The listing builds one solid part. Answer for the finished solid, in the listing's coordinates (mm). A direction names the side the tool comes from. Coordinates: 2 decimals unless noted, no trailing zeros. Loops run counter-clockwise (first coordinate to the right, second up) from the corner with the lowest first, then second, coordinate; pieces in that order, holes last. Notation, with made-up numbers: (65, -3.5) - (116, -3.5) arc R18 ccw to (116, 27.5) - close; hole circle Ø7 at (25.25, -4.75). An arc over 180 degrees is marked (long way). Write each question's results on one line, items separated by ' | '. Start each with the question number.
(1) Find section D-D on x = 4. Determine the outline of the cut face in (y, z).
(2) Find section C-C on x = 0. Determine the outline of the cut face in (y, z), then the cut area to 3 significant figures.
(3) Find section A-A on z = 6.5. Determine the outline of the cut face in (x, y).
(4) Consider line 1 (X direction, y = 9.75, z = 3.25); line 2 (Z direction, x = 2.5, y = -5.5); line 3 (Y direction, x = -9.5, z = 3.75). Determine where each line is inside the solid, lowest interval first. Write a range as from..to.
(5) Given pin 1 Ø6 at (y, z) = (7, 3.5) entering from +X; pin 2 Ø1.5 at (x, z) = (3, 5) entering from -Y; pin 3 Ø2.5 at (x, z) = (7, 5.5) entering from +Y, each flat-ended and moving along its own axis, determine where each tip first touches the part or whether it passes through.
(6) For faces 4 (the flat face through (-8, -0.585, 5)), 5 (the flat face through (0, -10.589, 3)), 6 (the cylindrical face through (2.307, -4.436, 7.395)), 7 (the flat face through (0.66, -8, 5)), 8 (the flat face through (-10, 0, 3)), determine the directions among +Z, -Z, +X, -X, +Y, -Y from which every point of the face is accessible in a straight line to the end or side of a thin tool.
(7) Determine the mould class of faces 1 (the cylindrical face through (11.923, 3.755, -0.986)), 2 (the flat face through (-8, 0.585, 5)), 3 (the flat face through (-0.66, 8, 5)) for opening direction X: released by +X, released by -X, zero draft, split by the parting line, or undercut.
from build123d import *

# Parameters (mm, degrees)
F0_R     = 5
F2_DEPTH = 15
F1_W     = 9.3396854261
F1_H     = 1.1709111985
F1_W_2   = 1.3206291478
F1_H_2   = 10.0037873136
F3_DEPTH = 12
F4_SIZE  = 4.99999
F5_R     = 12.5
F6_DEPTH = 2


# Not quite as in the source:
# - a fillet or chamfer is up to 0.001 mm smaller than in the source, because OpenCascade refuses the exact size


with BuildPart() as f2:
    # F0 (on Top) → F2 (new body)
    with BuildSketch(Plane.XY):
        Circle(F0_R)
    extrude(amount=F2_DEPTH)

    # F1 (on Top) → F3 (join)
    with BuildSketch(Plane.XY):
        with Locations((5.330157287, 0)):
            Rectangle(F1_W, F1_H)
        with Locations((-5.330157287, 0)):
            Rectangle(F1_W, F1_H)
        with Locations((0, 5.587349256)):
            Rectangle(F1_W_2, F1_H_2)
        with Locations((0, -5.587349256)):
            Rectangle(F1_W_2, F1_H_2)
    extrude(amount=F3_DEPTH)

    # F4 (size 5 in the source; OpenCascade refuses exactly that, so slightly less here)
    f4_edges = [f2.edges().sort_by_distance(p)[0] for p in [
        (0, 10.589243, 12),
        (10, 0, 12),
        (0, -10.589243, 12),
        (-10, 0, 12),
    ]]
    chamfer(f4_edges, length=F4_SIZE)

    # F5 (on Top) → F6 (join)
    with BuildSketch(Plane.XY):
        Circle(F5_R)
    extrude(amount=-F6_DEPTH)


solid = f2.part
Values:
1) outline: (-11.84, -2) - (11.84, -2) - (11.84, 0) - (3, 0) - (3, 15) - (-3, 15) - (-3, 0) - (-11.84, 0) - close
2) outline: (-12.5, -2) - (12.5, -2) - (12.5, 0) - (10.59, 0) - (10.59, 7) - (5.59, 12) - (5, 12) - (5, 15) - (-5, 15) - (-5, 12) - (-5.59, 12) - (-10.59, 7) - (-10.59, 0) - (-12.5, 0) - close | area: 309 mm²
3) outline: (-10, -0.59) - (-4.97, -0.59) arc R5 ccw to (-0.66, -4.96) - (-0.66, -10.59) - (0.66, -10.59) - (0.66, -4.96) arc R5 ccw to (4.97, -0.59) - (10, -0.59) - (10, 0.59) - (4.97, 0.59) arc R5 ccw to (0.66, 4.96) - (0.66, 10.59) - (-0.66, 10.59) - (-0.66, 4.96) arc R5 ccw to (-4.97, 0.59) - (-10, 0.59) - close
4) line 1: x = -0.66..0.66 | line 2: z = -2..0 | line 3: y = -0.59..0.59
5) pin 1: stops at x = 3 | pin 2: stops at y = -4.47 | pin 3: stops at y = 0.59
6) face 4: +Z, -X, -Y | face 5: +Z, +X, -X, -Y | face 6: +Z | face 7: +Z, +X, -Y | face 8: +Z, -X, +Y, -Y
7) face 1: split by the parting line | face 2: zero draft | face 3: released by -X
